Design review of the part built by this model. Coordinates are the model's own, in mm. A direction names the side the tool comes from. Round coordinates to 2 decimals unless told otherwise and drop trailing zeros. Loops run counter-clockwise (first coordinate to the right, second up) from the corner with the lowest first, then second, coordinate; pieces in that order, holes last. Notation, with made-up numbers: (-32.75, 57) - (-13.75, 57) arc R12 cw to (-13.75, 61) - close; hole circle Ø6 at (86, -30). An arc over 180 degrees is marked (long way). One line per question, with ' | ' between items. Start each with the question number.
from build123d import *

# Parameters (mm, degrees)
F0_R     = 11.402
F1_DEPTH = 74.6
F2_R     = 18.172457
F3_DEPTH = 11.9
F4_R     = 7.470799
F5_DEPTH = 67.4


with BuildPart() as f1:
    # F0 (on Front) → F1 (new body)
    with BuildSketch(Plane.XZ):
        with Locations((1.429774, 0)):
            Circle(F0_R)
    extrude(amount=F1_DEPTH)

    # F2 (on face) → F3 (join)
    with BuildSketch(Plane(origin=(0, 0, 0), x_dir=(-1, 0, 0), z_dir=(0, 1, 0))):
        with Locations((-1.429774, 0)):
            Circle(F2_R)
    extrude(amount=F3_DEPTH)

    # F4 (on face) → F5 (cut)
    with BuildSketch(Plane.XZ.offset(74.6)):
        with Locations((1.429774, 0)):
            Circle(F4_R)
    extrude(amount=-F5_DEPTH, mode=Mode.SUBTRACT)


solid = f1.part
1. Take a section at D-D, the plane x = 10. Give the boundary of the cut face in (y, z), then the cut area to 3 significant figures.
2. Machinability: for faces 1 (the face through (5.37, 5.87, -17.74)), 2 (the face through (10, 0, -8)), which of the approach directions +Z, -Z, +X, -X, +Y, -Y give a long, thin tool a straight path to every point of the face, cutting with its end or side? Answer none if there is none.
3. Clearance check with flat-ended pins moving along their axes: P1, Ø4.5, axis at x = 3, z = 1.5, coming from the -Y side; P2, Ø4, axis at y = -27.5, z = 7.5, coming from the +X side; P3, Ø5, axis at y = -31.5, z = -10, coming from the -X side. State where each tip first meets the part, or that it passes through.
4. Take a section at B-B, the plane y = -18. Give the boundary of the cut face in (x, z), then the cut area to 3 significant figures.
5. To check wall thickness, follow line 1 along Y through (x, z) = (13.5, 5.5); line 2 along Z through (x, y) = (1, -53); line 3 along Y through (x, z) = (4.5, 2.5). State the ranges of each line that lie inside material, in increasing order.
6. Take a section at C-C, the plane x = -4. Give the boundary of the cut face in (y, z).
7. Take a section at A-A, the plane z = 0. Give the boundary of the cut face in (x, y).
8. The part is to be moulded in two halves that separate along X. For faces 3 (the face through (12.305, -36.778, 3.425)), 4 (the face through (3.8, -74.6, -7.4)), 5 (the face through (1, -7.2, 0)), say which applies: pulls with the +X half, pulls with the -X half, needs draft (parallel to the pull), parting line crosses it, or undercut.
Answer list:
1) outline: (-74.6, -7.52) - (0, -7.52) - (0, -16.02) - (11.9, -16.02) - (11.9, 16.02) - (0, 16.02) - (0, 7.52) - (-74.6, 7.52) - close | area: 1,500 mm²
2) face 1: +Y, -Y | face 2: -Y
3) P1: stops at y = -7.2 | P2: stops at x = 11.42 | P3: stops at x = -7.16
4) outline: circle Ø22.8 at (1.43, 0); hole circle Ø14.94 at (1.43, 0) | area: 233 mm²
5) line 1: y = 0 to 11.9 | line 2: z = -11.39 to -7.46, 7.46 to 11.39 | line 3: y = -7.2 to 11.9
6) outline: (-74.6, -10.03) - (0, -10.03) - (0, -17.34) - (11.9, -17.34) - (11.9, 17.34) - (0, 17.34) - (0, 10.03) - (-74.6, 10.03) - (-74.6, 5.13) - (-7.2, 5.13) - (-7.2, -5.13) - (-74.6, -5.13) - close
7) outline: (-16.74, 0) - (-9.97, 0) - (-9.97, -74.6) - (-6.04, -74.6) - (-6.04, -7.2) - (8.9, -7.2) - (8.9, -74.6) - (12.83, -74.6) - (12.83, 0) - (19.6, 0) - (19.6, 11.9) - (-16.74, 11.9) - close
8) face 3: parting line crosses it | face 4: needs draft | face 5: undercut
